Input: part model. Units: mm. Frame: model coordinates. A direction names the side the tool comes from. Round coordinates to 2 decimals unless told otherwise and drop trailing zeros. Loops run counter-clockwise (first coordinate to the right, second up) from the corner with the lowest first, then second, coordinate; pieces in that order, holes last. Notation, with made-up numbers: (16.25, 66.25) -> (22.25, 66.25) arc R24 ccw to (22.25, 102.25) -> close; hole circle Ø5 at (44.25, 16.5). An arc over 180 degrees is marked (long way). Answer as a JSON object with one key per item and string values.
```python
from build123d import *

# Parameters (mm, degrees)
SKETCH1_R           = 2
SKETCH1_R_2         = 2.38125
SKETCH1_R_3         = 1.97
BASE_DEPTH          = 6
ALL_CUTS_DEPTH      = 76.612498967
ALL_CUTS_DEPTH_BACK = 76.612498967
SKETCH2_W           = 5
SKETCH2_H           = 30
SKETCH2_W_2         = 6
SKETCH2_H_2         = 20
SKETCH2_W_3         = 8
FILLET1_R           = 2.5


with BuildPart() as part:
    # Sketch1 → BASE (new, symmetric)
    with BuildSketch(Plane(origin=(0, 0, 0), x_dir=(0, 0, -1), z_dir=(1, 0, 0))):
        with BuildLine():
            Line((-67.5, 7.5), (67.5, 7.5))
            ThreePointArc((67.5, 7.5), (75, 0), (67.5, -7.5))
            Line((67.5, -7.5), (-67.5, -7.5))
            ThreePointArc((-67.5, -7.5), (-75, 0), (-67.5, 7.5))
        make_face()
        with Locations((-67.5, 0)):
            Circle(SKETCH1_R, mode=Mode.SUBTRACT)
        Circle(SKETCH1_R_2, mode=Mode.SUBTRACT)
        with Locations((67.5, 0)):
            Circle(SKETCH1_R_3, mode=Mode.SUBTRACT)
    extrude(amount=BASE_DEPTH, both=True)

    # Sketch2 → All_Cuts (cut, two sides: drawn at the far end of the back side and taken through both)
    with BuildSketch(Plane(origin=(0, 0, 0), x_dir=(1, 0, 0), z_dir=(0, 1, 0)).offset(-ALL_CUTS_DEPTH_BACK)):
        with Locations((0, -75)):
            Rectangle(SKETCH2_W, SKETCH2_H)
        with Locations((-6, -30)):
            Rectangle(SKETCH2_W_2, SKETCH2_H_2)
        with Locations((6, -30)):
            Rectangle(SKETCH2_W_2, SKETCH2_H_2)
        with Locations((6, 60)):
            Rectangle(SKETCH2_W_2, SKETCH2_H)
        with Locations((-6, 60)):
            Rectangle(SKETCH2_W_2, SKETCH2_H)
        Rectangle(SKETCH2_W_3, SKETCH2_H_2)
    extrude(amount=ALL_CUTS_DEPTH + ALL_CUTS_DEPTH_BACK, mode=Mode.SUBTRACT)

    # Fillet1
    fillet1_edges = [part.edges().sort_by_distance(p)[0] for p in [
        (3, 0, 20),
        (3, 0, 40),
        (-3, 0, 40),
        (-3, 0, 20),
        (3, 0, -45),
        (-3, 0, -45),
    ]]
    fillet(fillet1_edges, radius=FILLET1_R)


solid = part.part
```
1) Section C-C, the plane y = 0. Count the separate pieces of the cut face and the enclosed holes in it, plus the area to 3 significant figures.
Output:
{"separate pieces": "5", "enclosed holes": "0", "area": "1,200 mm^2"}
2) Contact query for flat-ended pins moving along their axis: P1, Ø2.5, axis at x = -0.5, y = -2, coming from the -Z side; P2, Ø0.6, axis at x = -5.5, y = -1, coming from the -Z side; P3, Ø5, axis at y = 0, z = -67.5, coming from the -X side; P4, Ø1, axis at x = 4, z = 24, coming from the -Y side. Output: stop coordinate, or through.
Output:
{"P1": "stops at z = -74.96", "P2": "stops at z = -45.02", "P3": "stops at x = -3", "P4": "passes through"}
3) Reachability of faces 4 (the face through (3, 0, 30)), 5 (the face through (3, 0, -61)), 6 (the face through (0, 0, -10)) from +Z, -Z, +X, -X, +Y, -Y: full face, straight path, thin tool, end or side. Return the list, or none.
Output:
{"face 4": "+X, +Y, -Y", "face 5": "-Z, +X, +Y, -Y", "face 6": "+Y, -Y"}
4) Section A-A, the plane x = 1. Output: boundary loops of the cut face in (y, z).
Output:
{"outline": "(-7.5, -67.5) arc R7.5 ccw to (7.5, -67.5) -> (7.5, -10) -> (-7.5, -10) -> close; (-7.5, 10) -> (7.5, 10) -> (7.5, 60) -> (-7.5, 60) -> close; hole circle Ø3.94 at (0, -67.5)"}
5) Section B-B, the plane z = -7. Output: boundary loops of the cut face in (x, y), plus the area to 3 significant figures.
Output:
{"outline": "(-6, -7.5) -> (-4, -7.5) -> (-4, 7.5) -> (-6, 7.5) -> close; (4, -7.5) -> (6, -7.5) -> (6, 7.5) -> (4, 7.5) -> close", "area": "60.0 mm^2"}
6) Ray query, probe 1 along Z at (x, y) = (0.1, 0); probe 2 along Z at (x, y) = (-5.5, 0); probe 3 along Z at (x, y) = (-4.25, 0). Return the intervals inside material, ascending.
Output:
{"probe 1": "z = -75 to -69.47, -65.53 to -10, 10 to 60", "probe 2": "z = -45 to -2.38, 2.38 to 20, 40 to 65.5, 69.5 to 75", "probe 3": "z = -45.33 to -2.38, 2.38 to 20.33, 39.67 to 65.5, 69.5 to 75"}
7) Draft query along Z for faces 1 (the face through (5, 7.5, 1)), 2 (the face through (4, 0, 75)), 3 (the face through (4, -2, 2)). Return one class per face: +Z half, -Z half, draft (parallel to the pull), parting line (faces both ways), or undercut.
Output:
{"face 1": "draft", "face 2": "+Z half", "face 3": "undercut"}
